Can you work these out from the drawing? Everything is in mm from the part's minimum corner. A direction names the side the tool comes from. Round coordinates to 2 decimals unless told otherwise and drop trailing zeros. Order: outer loops, then holes, each group sorted by start corner. A loop starts at its lowest first (then second) coordinate and runs counter-clockwise, first axis right, second up. Notation, with made-up numbers: M -37,49 L -21,49 A13 cw -21,62 Z; hole C 39.25,24 d1. An arc over 180 degrees is marked long. Answer as a JSON object with one key per item and string values. Group by question number.
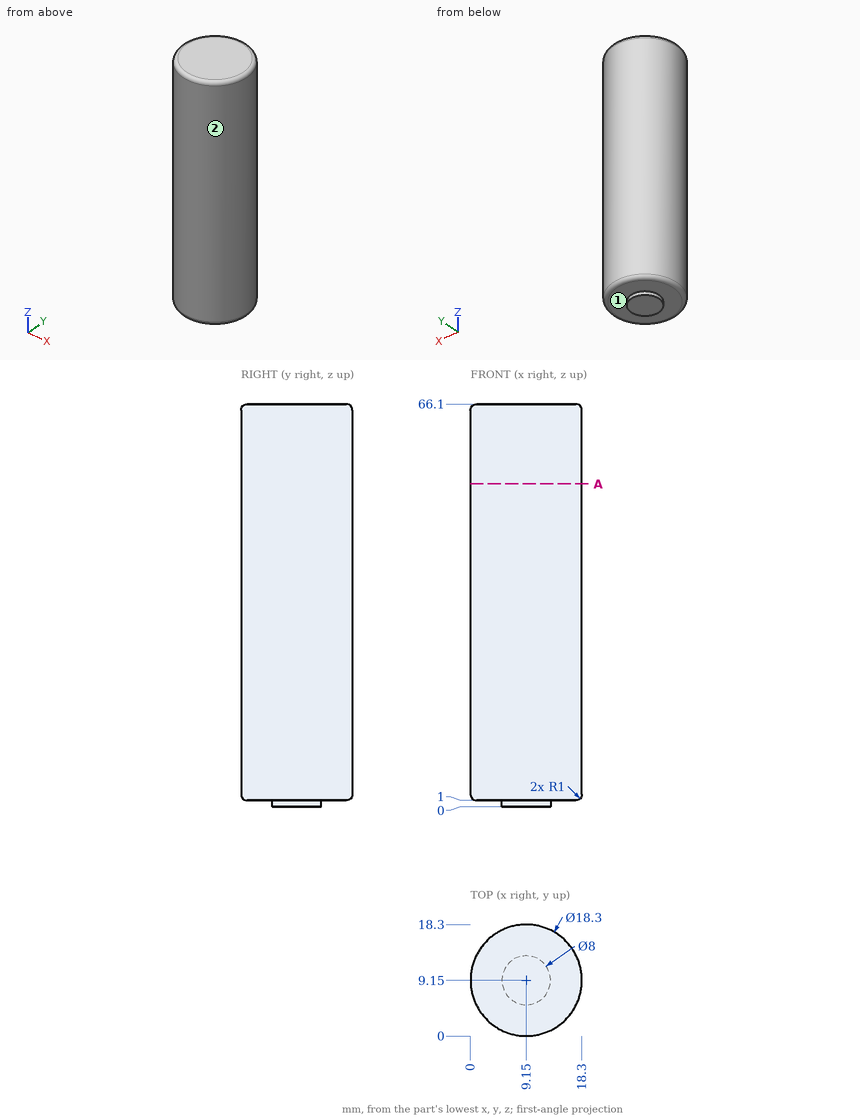
Item 1: I need wall thicknesses on line 1 (Z direction, x = 16.5, y = 5.25); line 2 (Y direction, x = 11.25, z = 58); line 3 (X direction, y = 13.5, z = 19.5). Which ranges of each line are inside material? Lowest first, please.
Item 2: On a 3-axis mill with a long thin cutter (end or side, diameter ignored), from which of +Z, -Z, +X, -X, +Y, -Y can I reach the whole of each face in a straight line? I mean the marked faces 1 and 2. Say none if no direction works.
Item 3: I'm going to push flat-ended pins straight in: pin 1 Ø1 at (x, y) = (3.5, 16) entering from -Z; pin 2 Ø2 at (x, z) = (11, 16) entering from -Y; pin 3 Ø5 at (y, z) = (2.5, 28.5) entering from +X. Where does each tip first touch, or does it pass through?
Item 4: Suppose I cut it at A-A, the plane z = 53. Write out the boundary of the cut face in (x, y).
Computed:
{
 "1": {"line 1": "z = 1.01 to 66.09", "line 2": "y = 0.24 to 18.06", "line 3": "x = 1.1 to 17.2"},
 "2": {"face 1": "-Z", "face 2": "+Z, -Z"},
 "3": {"pin 1": "stops at z = 1.03", "pin 2": "stops at y = 0.04", "pin 3": "stops at x = 17.3"},
 "4": {"outline": "C 9.15,9.15 d18.3"}
}
